Can you work these out from the drawing? Everything is in mm from the part's minimum corner. A direction names the side the tool comes from. Coordinates: 2 decimals unless noted, no trailing zeros. Order: outer loops, then holes, each group sorted by start corner. A loop starts at its lowest first (then second) coordinate and runs counter-clockwise, first axis right, second up. Notation, with made-up numbers: (78, -15.5) -> (129, -15.5) arc R24 ccw to (129, -1.5) -> close; hole circle Ø3 at (8.5, 58). An arc over 180 degrees is marked (long way). Answer in a Markdown table with one row per item.
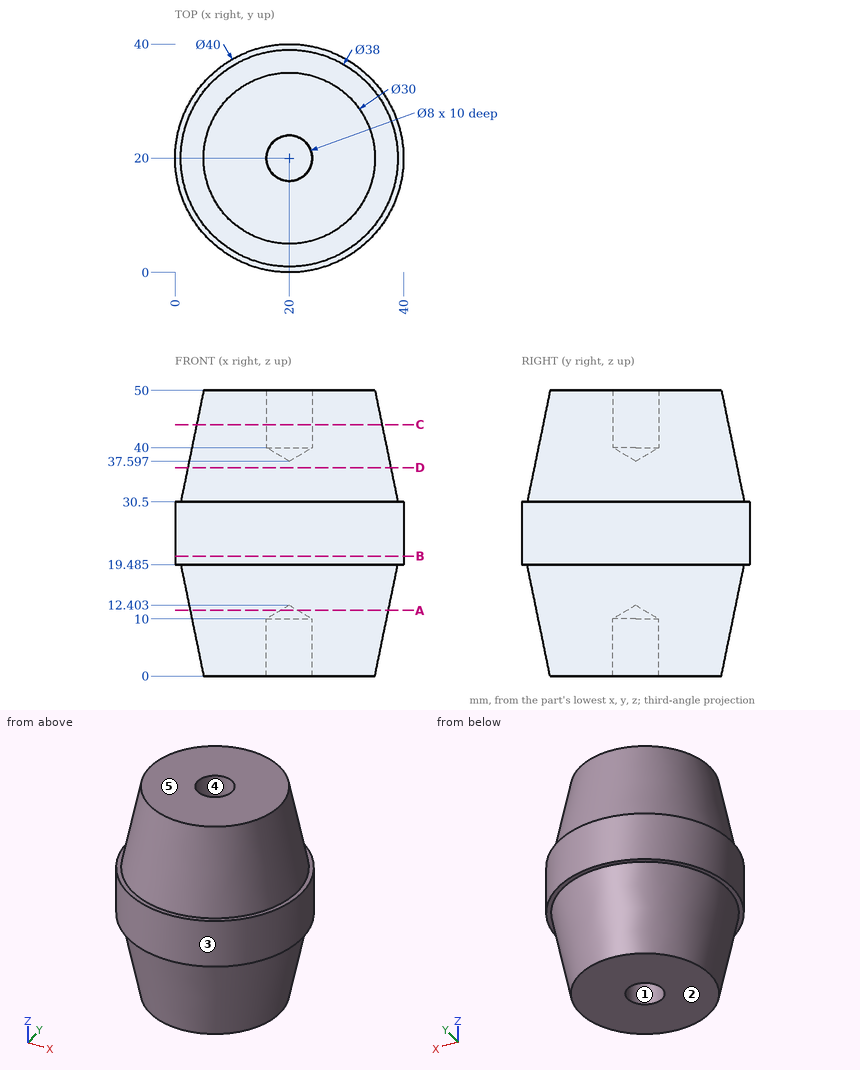
(1) Suppose I cut it at D-D (z = 36.5). Please give me the cut outline in (x, y), and give its area (3 significant figures).
Response values:
| item | result |
|---|---|
| outline | circle Ø35.54 at (20, 20) |
| area | 992 mm2 |
(2) Suppose I cut it at C-C (z = 44). Please give me the cut outline in (x, y).
Response values:
| item | result |
|---|---|
| outline | circle Ø32.46 at (20, 20); hole circle Ø8 at (20, 20) |
(3) I need wall thicknesses on line 1 (Y direction, x = 20, z = 7); line 2 (X direction, y = 20, z = 47) (1 decimal); line 3 (Z direction, x = 37.5, y = 12.5) (1 decimal). Which ranges of each line are inside material? Lowest first, please. Write a range as [from, to].
Response values:
| item | result |
|---|---|
| line 1 | [3.56, 16], [24, 36.44] |
| line 2 | [4.4, 16], [24, 35.6] |
| line 3 | [19.5, 30.5] |
(4) Suppose I cut it at A-A (z = 11.5). Please give me the cut outline in (x, y).
Response values:
| item | result |
|---|---|
| outline | circle Ø34.72 at (20, 20); hole circle Ø3.01 at (20, 20) |
(5) On a 3-axis mill with a long thin cutter (end or side, diameter ignored), from which of +Z, -Z, +X, -X, +Y, -Y can I reach the whole of each face in a straight line? I mean the marked faces 1 and 2. Say none if no direction works.
Response values:
| item | result |
|---|---|
| face 1 | -Z |
| face 2 | -Z, +X, -X, +Y, -Y |
(6) Suppose I cut it at B-B (z = 21). Please give me the cut outline in (x, y), and give its area (3 significant figures).
Response values:
| item | result |
|---|---|
| outline | circle Ø40 at (20, 20) |
| area | 1,260 mm2 |
(7) Will these pins go through, and if not, where does the flat tip stop? pin 1 Ø10 at (y, z) = (25.5, 28.5) entering from +X; pin 2 Ø1 at (y, z) = (24, 34) entering from +X; pin 3 Ø10 at (x, y) = (21, 23) entering from +Z; pin 4 Ø5 at (x, y) = (20, 20) entering from +Z.
Response values:
| item | result |
|---|---|
| pin 1 | x = 39.99 |
| pin 2 | x = 37.99 |
| pin 3 | z = 50 |
| pin 4 | z = 39.1 |
(8) We'd pull the mould along Y, two halves only. Please class the marked faces 3, 4 and 5: +Y half, -Y half, draft (parallel to the pull), parting line (faces both ways), or undercut.
Response values:
| item | result |
|---|---|
| face 3 | parting line |
| face 4 | undercut |
| face 5 | draft |
